The drawing under review shows one solid part. Ordinate dimensions are in mm from its lowest x, y, z. A direction names the side the tool comes from. Give positions to 0.01 mm unless a question says otherwise; leave off trailing zeros. Write each loop counter-clockwise with the first axis right and the second up, starting at its lowest first coordinate (ties: lowest second). Pieces come first, ordered by that corner, then holes.
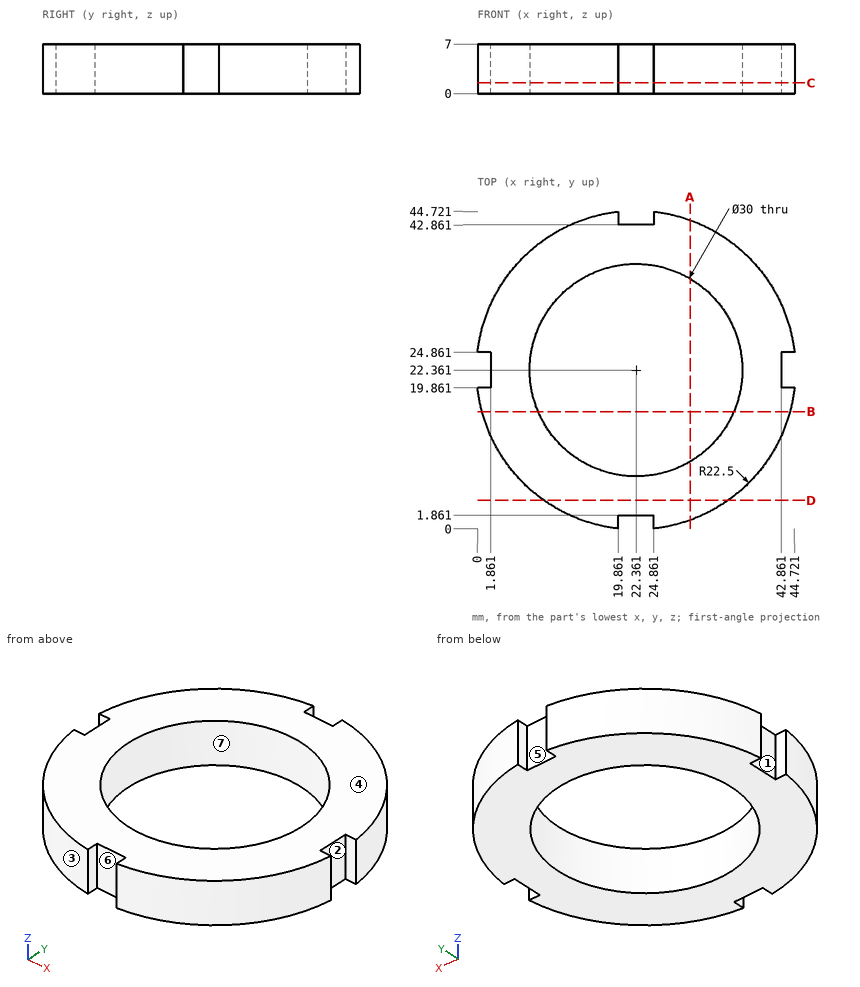
1) Consider section D-D, the plane y = 4. Give the boundary of the cut face in (x, z) (1 decimal).
2) To check wall thickness, follow probe 1 along Y at (x, z) = (33.5, 2.5) (1 decimal); probe 2 along Y at (x, z) = (22, 6.5) (1 decimal); probe 3 along X at (y, z) = (22.5, 5). State the ranges of each line that lie inside material, in increasing order.
3) Tool access review of the marked faces 5, 6 and 7: name each direction out of +Z, -Z, +X, -X, +Y, -Y from which nothing blocks a thin tool from reaching the whole face with its end or side.
4) Consider section B-B, the plane y = 16.5. Give the boundary of the cut face in (x, z).
5) The part is to be moulded in two halves that separate along Y. For the marked faces 1, 2, 3 and 4, say which applies: +Y half, -Y half, draft (parallel to the pull), parting line (faces both ways), or undercut.
6) Insertion check: pin 1 (12 mm diameter, centred on x = 7.5, y = 21, fed in from +Z); pin 2 (0.6 mm diameter, centred on y = 43.5, z = 2, fed in from +X) (1 decimal); pin 3 (3 mm diameter, centred on y = 34.5, z = 5, fed in from -X) (1 decimal); pin 4 (1.5 mm diameter, centred on y = 22.5, z = 5, fed in from +X). Each pin has a flat end and moves straight along its axis. Give the tip position at first contact, or say it passes through.
7) Consider section A-A, the plane x = 30. Give the boundary of the cut face in (y, z), then the cut area to 3 significant figures.
8) Consider section C-C, the plane z = 1.5. Give the boundary of the cut face in (x, y).
Answer block:
1. outline: (9.4, 0) - (35.4, 0) - (35.4, 7) - (9.4, 7) - close
2. probe 1: y = 2.8 to 12.3, 32.4 to 41.9
2. probe 2: y = 1.9 to 7.4, 37.4 to 42.9
2. probe 3: x = 1.86 to 7.36, 37.36 to 42.86
3. face 5: +Z, -Z, +Y
3. face 6: +Z, -Z, -Y
3. face 7: +Z, -Z
4. outline: (0.64, 0) - (8.55, 0) - (8.55, 7) - (0.64, 7) - close; (36.17, 0) - (44.08, 0) - (44.08, 7) - (36.17, 7) - close
5. face 1: undercut
5. face 2: undercut
5. face 3: -Y half
5. face 4: draft
6. pin 1: stops at z = 7
6. pin 2: stops at x = 30.8
6. pin 3: stops at x = 2.5
6. pin 4: stops at x = 42.86
7. outline: (1.2, 0) - (9.45, 0) - (9.45, 7) - (1.2, 7) - close; (35.27, 0) - (43.52, 0) - (43.52, 7) - (35.27, 7) - close
7. area: 116 mm2
8. outline: (0, 19.86) arc R22.5 ccw to (19.86, 0) - (19.86, 1.86) - (24.86, 1.86) - (24.86, 0) arc R22.5 ccw to (44.72, 19.86) - (42.86, 19.86) - (42.86, 24.86) - (44.72, 24.86) arc R22.5 ccw to (24.86, 44.72) - (24.86, 42.86) - (19.86, 42.86) - (19.86, 44.72) arc R22.5 ccw to (0, 24.86) - (1.86, 24.86) - (1.86, 19.86) - close; hole circle Ø30 at (22.36, 22.36)
